```python
from build123d import *

# Parameters (mm, degrees)
F0_R     = 3.175
F1_DEPTH = 25.4
F2_W     = 2.54
F2_H     = 1.5875
F3_DEPTH = 6.35
F4_R     = 2.53999


# Not quite as in the source:
# - a fillet or chamfer is up to 0.001 mm smaller than in the source, because OpenCascade refuses the exact size


with BuildPart() as f1:
    # F0 (on Top) → F1 (new body)
    with BuildSketch(Plane.XY):
        Circle(F0_R)
    extrude(amount=F1_DEPTH)

    # F2 (on face) → F3 (cut)
    with BuildSketch(Plane.XY.offset(25.4)):
        with Locations((1.905, 0)):
            Rectangle(F2_W, F2_H)
    extrude(amount=-F3_DEPTH, mode=Mode.SUBTRACT)

    # F4 (radius 2.54 in the source; OpenCascade refuses exactly that, so slightly less here)
    f4_edges = [f1.edges().sort_by_distance(p)[0] for p in [
        (0.635, 0, 19.05),
    ]]
    fillet(f4_edges, radius=F4_R)


solid = f1.part
```
Geometry check sheet. Reference: the model listing, model coordinates, mm. A direction names the side the tool comes from. Give positions to 0.01 mm unless a question says otherwise; leave off trailing zeros. Loops run counter-clockwise (first coordinate to the right, second up) from the corner with the lowest first, then second, coordinate; pieces in that order, holes last. Notation, with made-up numbers: M 69,49 L 116,49 A16 ccw 116,66 Z; hole C 18,18.25 d1. An arc over 180 degrees is marked long. Write item = value, one per line. Start each with the question number.
1. Thickness scan on probe 1 along Y at (x, z) = (1, 21); probe 2 along Y at (x, z) = (1.5, 19); probe 3 along Y at (x, z) = (-2, 6). Record the ranges inside material, lowest first.
2. Tool access check on faces 1 (the face through (1.399, 0.011, 19.774)), 2 (the face through (0, 0, 0)). Record the directions out of +Z, -Z, +X, -X, +Y, -Y that give a thin tool (end or side, any length) a straight path to the whole face; none if there is none.
3. Section check C-C, the plane y = -0.5. Enter the section's corners in (x, z) (3 decimals), plus the area to 3 significant figures.
4. Section check B-B, the plane z = 8.75. Enter the section's corners in (x, y) (3 decimals).
5. Section check D-D, the plane x = 2.5. Enter the section's corners in (y, z), plus the area to 3 significant figures.
6. Section check A-A, the plane x = 1.25. Enter the section's corners in (y, z).
7. Draft check along Y on faces 3 (the face through (2, -0.794, 22)), 4 (the face through (0, 0, 25.4)), 5 (the face through (-0.69, -3.1, 12.52)), 6 (the face through (2, 0.794, 22)). Enter one of: +Y half, -Y half, draft (parallel to the pull), parting line (faces both ways), or undercut.
8. Go/stop test with flat-tipped pins: P1, Ø1.2, axis at x = 2, z = 22, coming from the +Y side; P2, Ø1, axis at x = 1.5, z = 15, coming from the -Y side; P3, Ø1.3, axis at y = -0.5, z = 24.5, coming from the +X side. Record where each tip stops, or that it passes through.
Values follow:
q1.probe_1 = -3.01 to -0.79, 0.79 to 3.01
q1.probe_2 = -2.8 to 2.8
q1.probe_3 = -2.47 to 2.47
q2.face_1 = +Z, +X
q2.face_2 = -Z, +X, -X, +Y, -Y
q3.outline = M -3.135,0 L 3.135,0 L 3.135,19.05 A2.54 cw 0.635,21.59 L 0.635,25.4 L -3.135,25.4 Z
q3.area = 145 mm^2
q4.outline = C 0,0 d6.35
q5.outline = M -1.96,0 L 1.96,0 L 1.96,25.4 L 0.79,25.4 L 0.79,19.14 L -0.79,19.14 L -0.79,25.4 L -1.96,25.4 Z
q5.area = 89.5 mm^2
q6.outline = M -2.92,0 L 2.92,0 L 2.92,25.4 L 0.79,25.4 L 0.79,19.93 L -0.79,19.93 L -0.79,25.4 L -2.92,25.4 Z
q7.face_3 = undercut
q7.face_4 = draft
q7.face_5 = parting line
q7.face_6 = undercut
q8.P1 = 2.85
q8.P2 = -3.01
q8.P3 = 3.07
